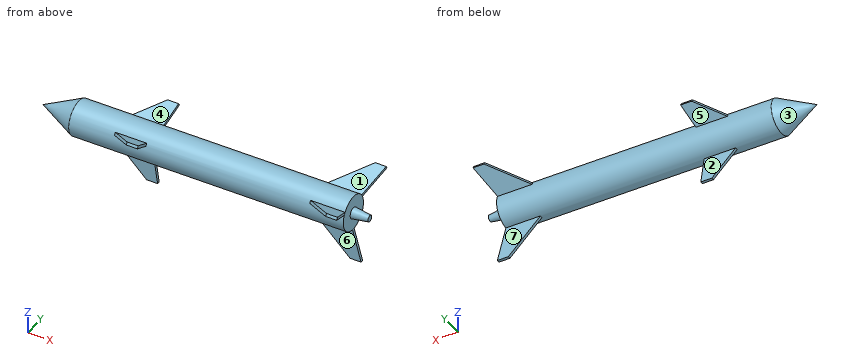
from build123d import *

# Parameters (mm, degrees)
RESSALTO_EXTRUS_O2_DEPTH = 1
RESSALTO_EXTRUS_O3_DEPTH = 1
PADR_OCIRCULAR2_COUNT    = 3
ESBO_O4_R                = 4
RESSALTO_EXTRUS_O4_DEPTH = 12
RESSALTO_EXTRUS_O4_TAPER = 8


with BuildPart() as part:
    # Esboço1 → Revolução1 (revolve)
    with BuildSketch(Plane.XY, mode=Mode.PRIVATE) as revolu_o1_sk:
        Polygon((0, 0), (26.038858788, 12.7), (226.038858788, 12.7), (226.038858788, 0), align=None)
    revolve(revolu_o1_sk.sketch.rotate(Axis((-90.349509161, 0, 0), (1, 0, 0)), 270), axis=Axis((-90.349509161, 0, 0), (1, 0, 0)))

    # Esboço3 → Ressalto-extrusão2 (add, symmetric)
    with BuildSketch(Plane(origin=(0, 0, 0), x_dir=(1, 0, 0), z_dir=(0, 1, 0))):
        Polygon((222.578858788, 0), (232.225029716, 36), (224.225029716, 36), (188.225029716, 0), align=None)
    ressalto_extrus_o2 = extrude(amount=RESSALTO_EXTRUS_O2_DEPTH, both=True)

    # Esboço2 → Ressalto-extrusão3 (add, symmetric)
    with BuildSketch(Plane(origin=(0, 0, 0), x_dir=(1, 0, 0), z_dir=(0, 1, 0))):
        Polygon((76.038858788, 30), (84.038858788, 30), (79.822633747, 0), (46.038858788, 0), align=None)
    ressalto_extrus_o3 = extrude(amount=RESSALTO_EXTRUS_O3_DEPTH, both=True)

    # PadrãoCircular2: Ressalto-extrusão2, Ressalto-extrusão3 ×3 about axis
    padr_ocircular2_axis = Axis((0, 0, 0), (1, 0, 0))
    add([ressalto_extrus_o2.rotate(padr_ocircular2_axis, i * 360 / PADR_OCIRCULAR2_COUNT) for i in range(1, PADR_OCIRCULAR2_COUNT)])
    add([ressalto_extrus_o3.rotate(padr_ocircular2_axis, i * 360 / PADR_OCIRCULAR2_COUNT) for i in range(1, PADR_OCIRCULAR2_COUNT)])

    # Esboço4 → Ressalto-extrusão4 (add)
    with BuildSketch(Plane(origin=(226.038858788, 0, 0), x_dir=(0, 0, -1), z_dir=(1, 0, 0))):
        Circle(ESBO_O4_R)
    extrude(amount=RESSALTO_EXTRUS_O4_DEPTH, taper=RESSALTO_EXTRUS_O4_TAPER)


solid = part.part
The listing builds one solid part. Answer for the finished solid, in the listing's coordinates (mm). Face numbers are marked on the shaded views. A direction names the side the tool comes from. Round coordinates to 2 decimals unless told otherwise and drop trailing zeros. Write each loop counter-clockwise with the first axis right and the second up, starting at its lowest first coordinate (ties: lowest second). Pieces come first, ordered by that corner, then holes. Notation, with made-up numbers: (-6, 22.5) - (39, 22.5) arc R13 cw to (39, 29.5) - close; hole circle Ø2 at (-40, 67). An arc over 180 degrees is marked (long way). Use a Markdown table: item, result. Add a question column.
1. Consider line 1 (Y direction, x = 218.5, z = 10.5); line 2 (Y direction, x = 202, z = 9.5); line 3 (Z direction, x = 100.5, y = 11.5). Determine where each line is inside the solid, lowest interval first.
2. The part is cut by section A-A (x = 217.5). Write down the section's boundary in (y, z), and give its area (3 significant figures).
3. For a pull along Y with two mould halves and no side action, classify the marked faces 1, 2 and 3 as +Y half, -Y half, draft (parallel to the pull), parting line (faces both ways), or undercut.
4. Flat-ended cylindrical pins translate along their axes: P1, Ø8, axis at x = 107.5, z = -7.5, coming from the +Y side; P2, Ø20.5, axis at y = 4.5, z = 0.5, coming from the +X side; P3, Ø2, axis at x = 78.5, y = 0.5, coming from the -Z side; P4, Ø11.5, axis at x = 213, z = -24, coming from the +Y side. Find the tip coordinate at first contact, or state that the pin passes through.
5. The part is cut by section B-B (x = 176.5). Write down the section's boundary in (y, z), and give its area (3 significant figures).
6. A tool of negligible diameter and unlimited length cuts with its end or side. For the marked faces 4, 5, 6 and 7, from which of +Z, -Z, +X, -X, +Y, -Y can it reach the whole face along a straight path? Write none if from no direction.
Reported:
| question | item | result |
|---|---|---|
| 1 | line 1 | -20.19 to -16.19, -7.14 to 7.14, 16.19 to 20.19 |
| 1 | line 2 | -8.43 to 8.43 |
| 1 | line 3 | -5.39 to 5.39 |
| 2 | outline | (-25.85, 13.77) - (-11.46, 5.46) arc R12.7 ccw to (-1, -12.66) - (-1, -29.27) - (1, -29.27) - (1, -12.66) arc R12.7 ccw to (11.46, 5.46) - (25.85, 13.77) - (24.85, 15.5) - (10.46, 7.2) arc R12.7 ccw to (-10.46, 7.2) - (-24.85, 15.5) - close |
| 2 | area | 606 mm^2 |
| 3 | face 1 | undercut |
| 3 | face 2 | +Y half |
| 3 | face 3 | parting line |
| 4 | P1 | y = 12.21 |
| 4 | P2 | x = 238.04 |
| 4 | P3 | z = -30 |
| 4 | P4 | y = 1 |
| 5 | outline | circle Ø25.4 at (0, 0) |
| 5 | area | 507 mm^2 |
| 6 | face 4 | +Z, +X, -X |
| 6 | face 5 | +X, -X, +Y |
| 6 | face 6 | -Z, +X, -X, -Y |
| 6 | face 7 | -Z, +X, -X, +Y |
